Autodesk Inventor part; units mm, degrees
ref_plane "YZ Plane" through (0, 0, 0) normal (1, 0, 0) x (0, 1, 0)
ref_plane "XZ Plane" through (0, 0, 0) normal (0, 1, 0) x (-1, 0, 0)
ref_plane "XY Plane" through (0, 0, 0) normal (0, 0, 1) x (1, 0, 0)
sketch "Sketch1" plane through (0, 0, 0) normal (0, 0, 1) x (1, 0, 0)
  circle A0 centre (50.8, 50.8) radius 2.54
  circle A1 centre (50.8, 38.1) radius 2.54
  line L0 (50.8, 57.15) -> (57.15, 57.15)
  line L1 (57.15, 57.15) -> (57.15, 50.8)
  line L2 (50.8, 57.15) -> (44.45, 57.15)
  line L3 (44.45, 57.15) -> (44.45, 31.75)
  line L4 (44.45, 31.75) -> (57.15, 31.75)
  circle A2 centre (0, 0) radius 2.54
  circle A3 centre (0, 25.4) radius 2.54
  line L5 (57.15, 50.8) -> (57.15, 31.75)
  line L6 (50.8, 38.1) -> (50.8, 44.45)
  line L7 (50.8, 38.1) -> (57.15, 31.75)
  line L8 (50.8, 38.1) -> (44.45, 44.45)
  line L9 (0, 0) -> (6.35, 0)
  line L10 (6.35, 0) -> (6.35, 31.75)
  line L11 (6.35, -6.35) -> (6.35, 0)
  line L12 (0, 0) -> (6.35, -6.35)
  line L13 (0, 25.4) -> (0, 31.75)
  line L14 (0, 31.75) -> (-3.9624, 31.75)
  line L15 (-3.9624, 31.75) -> (-3.9624, -6.35)
  line L16 (-3.9624, -6.35) -> (6.35, -6.35)
  line L17 (6.35, -6.35) -> (57.15, 31.75)
  line L18 (0, 0) -> (-6.358, 6.358)
  line L19 (49.0039, 39.8961) -> (-1.7961, 1.7961)
  line L20 (0, 31.75) -> (6.35, 31.75)
  point P0 (6.35, 7.9056)
  point P1 (44.45, 36.4806)
  dimension "d5" = 5.08
  dimension "d13" = 5.08
  dimension "d3" = 5.08
  dimension "d7" = 6.35
  dimension "d8" = 6.35
  dimension "d12" = 25.4
  dimension "d18" = 5.08
  dimension "d24" = 6.35
  dimension "d29" = 3.9624
  dimension "d30" = 8.9916
extrude "Extrusion1" add sketch "Sketch1" along normal blind 1.5875 contours A1 L8 L3 L2 L0 L1 L5 L7 | L7 L4 L3 L19 A1 | L19 L3 L8 | L17 L11 L10 L19 L3 L4 | L12 A2 L9 L11 | L16 L15 L18 A2 L12 | L19 A2 L18 L15 L14 L20 L10 | L10 L9 A2 L19
fillet "Fillet1" radius 3.175 9 edges at (44.45, 57.15, 0.7937) (57.15, 57.15, 0.7937) (57.15, 31.75, 0.7937) (44.45, 36.4806, 0.7937) (6.35, 7.9056, 0.7937) (6.35, 31.75, 0.7937) (-3.9624, 31.75, 0.7937) (-3.9624, -6.35, 0.7937) (6.35, -6.35, 0.7937)
properties part number "funnelPoly"
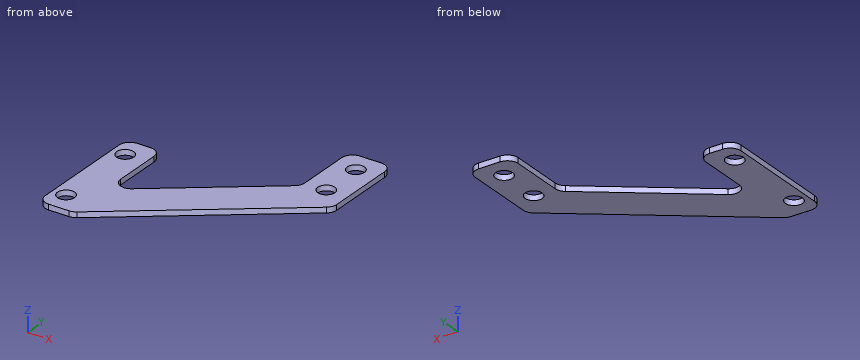
Here's how the part is built. I have some questions about the finished solid (model axes, mm). Give positions to 0.01 mm unless a question says otherwise; leave off trailing zeros. Write each loop counter-clockwise with the first axis right and the second up, starting at its lowest first coordinate (ties: lowest second). Pieces come first, ordered by that corner, then holes.
(1) Will these pins go through, and if not, where does the flat tip stop? pin 1 (6 mm diameter, centred on x = 0, y = 0, fed in from +Z); pin 2 (0.5 mm diameter, centred on y = 20, z = 0.5, fed in from +X); pin 3 (0.5 mm diameter, centred on y = 44, z = 0.5, fed in from -X).
Output values:
pin 1: stops at z = 1.59
pin 2: stops at x = 41.82
pin 3: stops at x = 44.45
(2) If I drill on L1, parallel to Y at x = 50.8, z = 0.6; L2, parallel to Y at x = 50, z = 1.45; L3, parallel to X at y = 44.5, z = 0.3, over which ranges is the centre line in solid material (lowest first)?
Output values:
L1: y = 26.99 to 35.56, 40.64 to 48.26, 53.34 to 57.15
L2: y = 26.39 to 35.69, 40.51 to 48.39, 53.21 to 57.15
L3: x = 44.45 to 57.15
(3) Imagine slicing it at A-A, the plane x = 0. Write out the boundary of the cut face in (y, z).
Output values:
outline: (-6.35, 0) - (-2.54, 0) - (-2.54, 1.59) - (-6.35, 1.59) - close; (2.54, 0) - (22.86, 0) - (22.86, 1.59) - (2.54, 1.59) - close; (27.94, 0) - (31.75, 0) - (31.75, 1.59) - (27.94, 1.59) - close
(4) Imagine slicing it at D-D, the plane y = 25.4. Write out the boundary of the cut face in (x, z), and give its area (3 significant figures).
Output values:
outline: (-3.96, 0) - (-2.54, 0) - (-2.54, 1.59) - (-3.96, 1.59) - close; (2.54, 0) - (6.35, 0) - (6.35, 1.59) - (2.54, 1.59) - close; (29.68, 0) - (48.68, 0) - (48.68, 1.59) - (29.68, 1.59) - close
area: 38.5 mm2
(5) Imagine slicing it at B-B, the plane y = 50.8. Write out the boundary of the cut face in (x, z).
Output values:
outline: (44.45, 0) - (48.26, 0) - (48.26, 1.59) - (44.45, 1.59) - close; (53.34, 0) - (57.15, 0) - (57.15, 1.59) - (53.34, 1.59) - close
(6) Imagine slicing it at C-C, the plane z = 1.1. Count the separate pieces of the cut face and the enclosed holes in it, and give its area (3 significant figures).
Output values:
separate pieces: 1
enclosed holes: 4
area: 1,240 mm2
